Check sheet for the modelled part. Datum: model origin and axes. Units: mm. A direction names the side the tool comes from. Round coordinates to 2 decimals unless told otherwise and drop trailing zeros. Write each loop counter-clockwise with the first axis right and the second up, starting at its lowest first coordinate (ties: lowest second). Pieces come first, ordered by that corner, then holes. Notation, with made-up numbers: (-21, 84) -> (-3, 84) arc R14 cw to (-3, 107) -> close; hole circle Ø5 at (38.25, 79.25). An arc over 180 degrees is marked (long way). One line per item, written item: value. Start each with the question number.
```python
from build123d import *


with BuildPart() as part:
    # Croquis1 → Revolución1 (revolve)
    with BuildSketch(Plane.XY, mode=Mode.PRIVATE) as revoluci_n1_sk:
        with BuildLine():
            Line((23.843190864, 18), (21.641499939, 18))
            Line((21.641499939, 18), (20.877394398, 19.095222917))
            ThreePointArc((20.877394398, 19.095222917), (20.232592167, 19.507553513), (19.485086377, 19.343171243))
            Line((19.485086377, 19.343171243), (17.559865516, 18))
            Line((17.559865516, 18), (12.843190864, 18))
            Line((12.843190864, 18), (12.843190864, 16.782184677))
            Line((12.843190864, 16.782184677), (15.239734897, 14.672192861))
            ThreePointArc((15.239734897, 14.672192861), (15.397557992, 14.189058917), (15.050891885, 13.817374713))
            Line((15.050891885, 13.817374713), (12.843190864, 13.165654901))
            Line((12.843190864, 13.165654901), (12.843190864, 12.5))
            Line((12.843190864, 12.5), (23.843190864, 12.5))
            Line((23.843190864, 12.5), (23.843190864, 13.017083416))
            Line((23.843190864, 13.017083416), (22.414504066, 13.535357634))
            ThreePointArc((22.414504066, 13.535357634), (22.221515959, 13.764442451), (22.32291652, 14.046297359))
            Line((22.32291652, 14.046297359), (23.843190864, 15.333938712))
            Line((23.843190864, 15.333938712), (23.843190864, 18))
        make_face()
    revolve(revoluci_n1_sk.sketch.rotate(Axis((29.11578235, 0, 0), (-1, 0, 0)), 90), axis=Axis((29.11578235, 0, 0), (-1, 0, 0)))


solid = part.part
```
1. Release check for a two-part mould opening along Z. For faces 3 (the face through (13, -0.6, 13.2)), 4 (the face through (15.12, 13.11, -6.82)), 5 (the face through (23.843, -8.1, 13.2)), 6 (the face through (15.169, -12.165, 13.267)) record: +Z half, -Z half, draft (parallel to the pull), parting line (faces both ways), or undercut.
2. Cross-section at D-D (x = 18.5). Record the cut outline in (y, z), plus the area to 3 significant figures.
3. Material ranges on probe 1 along Z at (x, y) = (22.5, 8.5); probe 2 along Y at (x, z) = (13.75, -5); probe 3 along Y at (x, z) = (13.5, -2.5), recorded low to high.
4. Access from +Z, -Z, +X, -X, +Y, -Y to the whole of each face (thin tool, end or side, straight path). Record for faces 1 (the face through (22.727, -12.165, 13.267)), 2 (the face through (12.843, 5, -12)).
5. Depth check by flat-ended pin: pin 1 Ø6 at (y, z) = (13.5, -5) entering from -X; pin 2 Ø1.5 at (x, y) = (22, 8.5) entering from +Z; pin 3 Ø3 at (x, z) = (19.5, 1.5) entering from +Y; pin 4 Ø2 at (x, z) = (16.5, -6.5) entering from -Y. Enter the tip coordinate at first touch or a pass-through.
6. Cross-section at C-C (x = 14.25). Record the cut outline in (y, z).
Working result:
1. face 3: undercut
1. face 4: undercut
1. face 5: draft
1. face 6: parting line
2. outline: circle Ø37.31 at (0, 0); hole circle Ø25 at (0, 0)
2. area: 603 mm^2
3. probe 1: z = -15.87 to -11.37, -10.49 to -9.17, 9.17 to 10.49, 11.37 to 15.87
3. probe 2: y = -17.29 to -15.18, -12.47 to -11.46, 11.46 to 12.47, 15.18 to 17.29
3. probe 3: y = -17.83 to -16.01, -13.12 to -12.25, 12.25 to 13.12, 16.01 to 17.83
4. face 1: +X
4. face 2: +Z, -Z, -X, +Y, -Y
5. pin 1: stops at x = 12.84
5. pin 2: stops at z = 16.56
5. pin 3: stops at y = 19.52
5. pin 4: stops at y = -17.14
6. outline: circle Ø36 at (0, 0); circle Ø27.16 at (0, 0); hole circle Ø31.09 at (0, 0); hole circle Ø25 at (0, 0)
